Autodesk Inventor part; units mm, degrees
ref_plane "YZ Plane" through (0, 0, 0) normal (1, 0, 0) x (0, 1, 0)
ref_plane "XZ Plane" through (0, 0, 0) normal (0, 1, 0) x (-1, 0, 0)
ref_plane "XY Plane" through (0, 0, 0) normal (0, 0, 1) x (1, 0, 0)
sketch "Sketch1" plane through (0, 0, 0) normal (0, 0, 1) x (1, 0, 0)
  line L0 (-3.8891, 0) -> (0, -3.8891)
  line L1 (0, -3.8891) -> (3.8891, 0)
  line L2 (3.8891, 0) -> (0, 3.8891)
  line L3 (0, 3.8891) -> (-3.8891, 0)
  line L4 (-3.8891, 0) -> (3.8891, 0) construction
  line L5 (0, -3.8891) -> (0, 3.8891) construction
  point P0 (0, 0)
  dimension "d0" = 5.5
  dimension "d1" = 5.5
  dimension "d2" = 90
  dimension "d3" = 5.5
  dimension "d4" = 90
  dimension "d5" = 0
  dimension "d6" = 0
extrude "Extrusion1" add sketch "Sketch1" along normal blind 3
sketch "Sketch2" plane through (0, 0, 0) normal (1, 0, 0) x (0, 1, 0)
  line L0 (3.8891, 0) -> (0, 0)
  line L1 (3.8891, 0) -> (3.8891, 0.75)
  line L2 (3.8891, 0.75) -> (3.1391, 0)
  line L3 (3.8891, 0) -> (3.1391, 0)
  line L4 (-3.8891, 3) -> (0, 3)
  line L5 (0, 3) -> (0, 0)
  dimension "d9" = 0.75
  dimension "d10" = 0.75
revolve "Revolution1" cut sketch "Sketch2" angle 360 about axis through (0, 0, 3) along (0, 0, -1)
sketch "Sketch3" plane through (0, 0, 3) normal (0, 0, 1) x (1, 0, 0)
  circle A0 centre (0, 0) radius 2.15
  dimension "d12" = 4.3
extrude "Extrusion2" add sketch "Sketch3" along normal blind 56
chamfer "Chamfer1" distance 1 angle 45 1 edges at (-2.15, 0, 59)
thread "Thread1"
properties part number "ES117_Bolt" material "Stainless Steel"
The listing builds one solid part. Answer for the finished solid, in the listing's coordinates (mm). A direction names the side the tool comes from. Coordinates: 2 decimals unless noted, no trailing zeros. Write each loop counter-clockwise with the first axis right and the second up, starting at its lowest first coordinate (ties: lowest second). Pieces come first, ordered by that corner, then holes.
Q1. Given P1, Ø1, axis at y = 0, z = 24, coming from the +X side; P2, Ø3, axis at x = -1.5, z = 33.5, coming from the +Y side; P3, Ø4, axis at y = 1.5, z = 26.5, coming from the -X side, each flat-ended and moving along its own axis, determine where each tip first touches the part or whether it passes through.
Returned:
P1: stops at x = 2.15
P2: stops at y = 2.15
P3: stops at x = -2.15
Q2. Section A-A, the plane z = 8.5 is taken. Write down the section's boundary in (x, y), then the cut area to 3 significant figures.
Returned:
outline: circle Ø4.3 at (0, 0)
area: 14.5 mm2
Q3. Which of the six approach directions +Z, -Z, +X, -X, +Y, -Y give full straight-line access (tool end or side, diameter ignored) to faces 1 (the flat face through (1.97, 1.92, 1.48)), 2 (the cylindrical face through (-2.15, -0.09, 30.12))?
Returned:
face 1: +Z, -Z, +X, +Y
face 2: +Z
Q4. Find the intervals of material crossed by line 1 along Z through (x, y) = (-1.5, -2); line 2 along Y through (x, z) = (1, 22); line 3 along X through (y, z) = (-0.25, 23), in increasing order.
Returned:
line 1: z = 0 to 3
line 2: y = -1.9 to 1.9
line 3: x = -2.14 to 2.14
